from build123d import *

# Parameters (mm, degrees)
F4_DEPTH = 20


with BuildPart() as f1:
    # F0 (on Front) → F1 (revolve)
    with BuildSketch(Plane.XZ):
        with BuildLine():
            ThreePointArc((-7.5, 0), (-5.732233, 0.732233), (-5, 2.5))
            ThreePointArc((-5, 2.5), (-5.336434, 3.752591), (-6.255187, 4.66805))
            ThreePointArc((-6.255187, 4.66805), (-9.915587, 3.144157), (-7.5, 0))
        make_face()
        with BuildLine():
            ThreePointArc((-6.255187, 4.66805), (-5.336434, 3.752591), (-5, 2.5))
            ThreePointArc((-5, 2.5), (-5.732233, 0.732233), (-7.5, 0))
            Line((-7.5, 0), (0, 0))
            Line((0, 0), (0, 3))
            ThreePointArc((0, 3), (-3.236887, 3.424174), (-6.255187, 4.66805))
        make_face()
    revolve(axis=Axis((0, 0, 1.5), (0, 0, 1)))

    # F3 (on offset) → F4 (cut)
    with BuildSketch(Plane.XY.offset(15)):
        Polygon((4.653195, 0.459226), (4.640465, 0.472158), (0.2023, 4.910323), (0.181042, 4.931338), (0.100782, 4.977652), (-0.014517, 5), (-0.129855, 4.977652), (-0.209914, 4.931338), (-0.230929, 4.910323), (-2.329216, 2.812076), (-2.34328, 2.798255), (-2.370195, 2.741676), (-2.371327, 2.664285), (-2.335804, 2.595664), (-2.286459, 2.557069), (-2.267586, 2.550684), (4.524479, 0.284722), (4.541776, 0.279024), (4.602113, 0.286258), (4.656468, 0.332491), (4.673806, 0.402001), align=None)
        Polygon((-2.337986, -2.803504), (-2.323963, -2.817536), (-0.230929, -4.910542), (-0.210116, -4.93137), (-0.129855, -4.977635), (-0.014517, -5), (0.100782, -4.977635), (0.181285, -4.931593), (0.2023, -4.910542), (4.639616, -0.473266), (4.652508, -0.460333), (4.672917, -0.402866), (4.65562, -0.333396), (4.601224, -0.287123), (4.540927, -0.279889), (4.52359, -0.285789), (-2.262333, -2.556398), (-2.281165, -2.562541), (-2.330752, -2.601128), (-2.366033, -2.669757), (-2.364942, -2.746934), align=None)
        Polygon((-0.987138, -0.125309), (-0.987138, 0.000982), (-0.987138, 0.127515), (-1.034704, 0.506792), (-1.163218, 0.95077), (-1.352392, 1.334937), (-1.581291, 1.661192), (-1.829509, 1.931313), (-2.076433, 2.147281), (-2.301372, 2.31063), (-2.437039, 2.396791), (-2.483352, 2.4231), (-2.505458, 2.43579), (-2.625646, 2.451389), (-2.737227, 2.40552), (-2.755211, 2.387334), (-4.924747, 0.217596), (-4.945802, 0.196581), (-4.992277, 0.116523), (-5.014626, 0.001225), (-4.992277, -0.114114), (-4.946045, -0.194375), (-4.924747, -0.215632), (-2.752786, -2.387573), (-2.734802, -2.405553), (-2.622777, -2.451377), (-2.502629, -2.43581), (-2.480483, -2.423092), (-2.43425, -2.396346), (-2.298745, -2.309959), (-2.07425, -2.146173), (-1.827771, -1.929992), (-1.579998, -1.659648), (-1.351583, -1.332961), (-1.162976, -0.948604), (-1.034502, -0.504384), align=None)
    extrude(amount=-F4_DEPTH, mode=Mode.SUBTRACT)


solid = f1.part
The listing builds one solid part. Answer for the finished solid, in the listing's coordinates (mm). Give positions to 0.01 mm unless a question says otherwise; leave off trailing zeros.
Item 1: Find the intervals of material crossed by line 1 along Y through (x, z) = (2.5, 1.2); line 2 along Y through (x, z) = (2, 2.35); line 3 along X through (y, z) = (4.5, 3.45), in increasing order.
Item 2: Determine the mould class of faces 1 (the flat face through (1.178, -1.405, 1.523)), 2 (the flat face through (0, 0, 0)) for opening direction Y: released by +Y, released by -Y, zero draft, split by the parting line, or undercut.
Item 3: Flat-ended cylindrical pins translate along their axes: P1, Ø2, axis at x = 0.5, z = 3.5, coming from the -Y side; P2, Ø3, axis at y = 0.5, z = 0.5, coming from the -X side; P3, Ø2, axis at x = -2, z = 3.5, coming from the +Y side. Find the tip coordinate at first contact, or state that the pin passes through.
Item 4: Section A-A, the plane x = 4.25 is taken. Count the separate pieces of the cut face and the enclosed holes in it, plus the area to 3 significant figures.
Completed:
1. line 1: y = -9.31 to -2.61, -0.96 to 0.96, 2.61 to 9.31
1. line 2: y = -9.79 to -3.11, -1.13 to 1.13, 3.11 to 9.79
1. line 3: x = -8.72 to -0.64, 0.61 to 8.72
2. face 1: undercut
2. face 2: zero draft
3. P1: stops at y = -10
3. P2: stops at x = -9.94
3. P3: stops at y = 9.9
4. separate pieces: 3
4. enclosed holes: 0
4. area: 71.7 mm2
